Verification items for the finished model (mm, model axes). A direction names the side the tool comes from. Round coordinates to 2 decimals unless told otherwise and drop trailing zeros. Loops run counter-clockwise (first coordinate to the right, second up) from the corner with the lowest first, then second, coordinate; pieces in that order, holes last.
from build123d import *

# Parameters (mm, degrees)
F0_W     = 50
F0_H     = 200
F1_DEPTH = 10
F2_R     = 3
F3_DEPTH = 25
F5_DEPTH = 25
F6_W     = 10
F6_H     = 10
F7_DEPTH = 10


with BuildPart() as f1:
    # F0 (on Front) → F1 (new body)
    with BuildSketch(Plane.XZ):
        Rectangle(F0_W, F0_H)
    extrude(amount=F1_DEPTH)

    # F2 (on face) → F3 (cut)
    with BuildSketch(Plane.XZ.offset(10)):
        with Locations((0, -25)):
            Circle(F2_R)
    extrude(amount=-F3_DEPTH, mode=Mode.SUBTRACT)

    # F4 (on face) → F5 (cut)
    with BuildSketch(Plane.XZ.offset(10)):
        with BuildLine():
            Line((10, 50), (-10, 50))
            Line((-10, 50), (-10, 30))
            ThreePointArc((-10, 30), (-8.5, 28.5), (-7, 30))
            Line((-7, 30), (7, 30))
            ThreePointArc((7, 30), (8.5, 28.5), (10, 30))
            Line((10, 30), (10, 50))
        make_face()
    extrude(amount=-F5_DEPTH, mode=Mode.SUBTRACT)

    # F6 (on face) → F7 (join)
    with BuildSketch(Plane.XZ.offset(10)):
        with Locations((-30, 65)):
            Rectangle(F6_W, F6_H)
        with Locations((30, 65)):
            Rectangle(F6_W, F6_H)
        with Locations((-30, -5)):
            Rectangle(F6_W, F6_H)
        with Locations((30, -5)):
            Rectangle(F6_W, F6_H)
    extrude(amount=-F7_DEPTH)


solid = f1.part
1. Section check A-A (x = 27). Enter the section's corners in (y, z), then the cut area to 3 significant figures.
2. Scan lines: L1, parallel to Z at x = 0, y = -1.75; L2, parallel to Z at x = 8.5, y = -7; L3, parallel to Z at x = 3.5, y = -5.25. Record each from-to range of solid material in increasing order.
3. Gauge pin test, flat ends, axial feed: P1, Ø3, axis at y = -4.5, z = 18, coming from the +X side; P2, Ø5, axis at x = -31.5, y = -6.5, coming from the -Z side; P3, Ø5, axis at y = -3, z = 15.5, coming from the -X side. Record the tip position at first contact, or that the pin passes through.
4. Section check C-C (x = 0). Enter the section's corners in (y, z), then the cut area to 3 significant figures.
5. Section check D-D (y = -7.75). Enter the section's corners in (x, z).
6. Section check B-B (z = -25). Enter the section's corners in (x, y).
7. Tool access check on faces 1 (the face through (-30, -5, 60)), 2 (the face through (0, -5, 50)), 3 (the face through (30, -5, 0)), 4 (the face through (-25, -5, -56)). Record the directions out of +Z, -Z, +X, -X, +Y, -Y that give a thin tool (end or side, any length) a straight path to the whole face; none if there is none.
8. Release check for a two-part mould opening along Z. For faces 5 (the face through (-35, -5, -5)), 6 (the face through (-30, -5, 70)), 7 (the face through (-10, -5, 40)) record: released by +Z, released by -Z, zero draft, split by the parting line, or undercut.
Taken from the geometry:
1. outline: (-10, -10) - (0, -10) - (0, 0) - (-10, 0) - close; (-10, 60) - (0, 60) - (0, 70) - (-10, 70) - close
1. area: 200 mm2
2. L1: z = -100 to -28, -22 to 30, 50 to 100
2. L2: z = -100 to 28.5, 50 to 100
2. L3: z = -100 to 30, 50 to 100
3. P1: stops at x = 25
3. P2: stops at z = -10
3. P3: stops at x = -25
4. outline: (-10, -100) - (0, -100) - (0, -28) - (-10, -28) - close; (-10, -22) - (0, -22) - (0, 30) - (-10, 30) - close; (-10, 50) - (0, 50) - (0, 100) - (-10, 100) - close
4. area: 1,740 mm2
5. outline: (-35, -10) - (-25, -10) - (-25, -100) - (25, -100) - (25, -10) - (35, -10) - (35, 0) - (25, 0) - (25, 60) - (35, 60) - (35, 70) - (25, 70) - (25, 100) - (-25, 100) - (-25, 70) - (-35, 70) - (-35, 60) - (-25, 60) - (-25, 0) - (-35, 0) - close; hole (-10, 30) arc R1.5 ccw to (-7, 30) - (7, 30) arc R1.5 ccw to (10, 30) - (10, 50) - (-10, 50) - close; hole circle Ø6 at (0, -25)
6. outline: (-25, -10) - (-3, -10) - (-3, 0) - (-25, 0) - close; (3, -10) - (25, -10) - (25, 0) - (3, 0) - close
7. face 1: -X, +Y, -Y
7. face 2: +Y, -Y
7. face 3: +X, +Y, -Y
7. face 4: -Z, -X, +Y, -Y
8. face 5: zero draft
8. face 6: released by +Z
8. face 7: undercut
